Geometry check sheet. Reference: the model listing, model coordinates, mm. Face numbers are marked on the shaded views. A direction names the side the tool comes from. Give positions to 0.01 mm unless a question says otherwise; leave off trailing zeros. Loops run counter-clockwise (first coordinate to the right, second up) from the corner with the lowest first, then second, coordinate; pieces in that order, holes last. Notation, with made-up numbers: (-11, 85.25) -> (-7, 85.25) arc R34 cw to (-7, 120.25) -> close; hole circle Ø3 at (23, 60.25). An arc over 180 degrees is marked (long way). One line per question, with ' | ' between items.
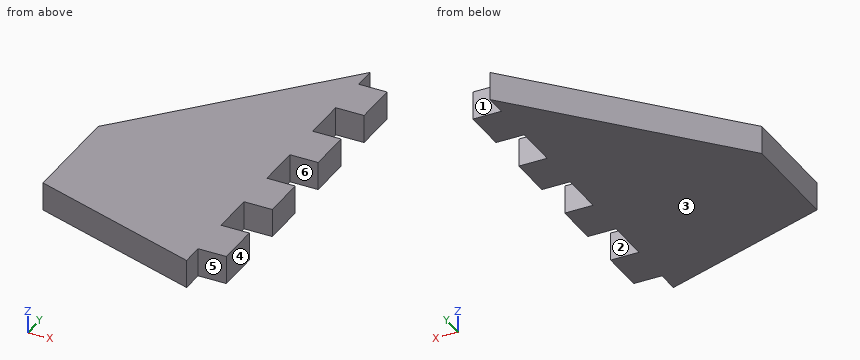
from build123d import *

# Parameters (mm, degrees)
ESTRUSIONE_ESTRUSIONE1_DEPTH = 4
SCHIZZO2_W                   = 4
SCHIZZO2_H                   = 6.25
ESTRUSIONE_ESTRUSIONE2_DEPTH = 4
RIPETIZIONE_A_L1_COUNT       = 4
RIPETIZIONE_A_L1_PITCH       = 12.5


with BuildPart() as part:
    # Schizzo1 → Estrusione-Estrusione1 (new body)
    with BuildSketch(Plane.XY):
        Polygon((-24.4, 23), (-24.4, 8), (0, 0), (0, 50), align=None)
    extrude(amount=ESTRUSIONE_ESTRUSIONE1_DEPTH)

    # Schizzo2 → Estrusione-Estrusione2 (add)
    with BuildSketch(Plane.XY.offset(4)):
        with Locations((2, 43.75)):
            Rectangle(SCHIZZO2_W, SCHIZZO2_H)
    estrusione_estrusione2 = extrude(amount=-ESTRUSIONE_ESTRUSIONE2_DEPTH)

    # Ripetizione a L1: Estrusione-Estrusione2 ×4
    with Locations(*[(0, -i * RIPETIZIONE_A_L1_PITCH, 0) for i in range(1, RIPETIZIONE_A_L1_COUNT)]):
        add(estrusione_estrusione2)


solid = part.part
Item 1: Set-up check for the marked faces 1, 2 and 3: record each of +Z, -Z, +X, -X, +Y, -Y from which the full face is reachable in a straight line by a thin tool's end or side.
Result:
face 1: +Z, -Z, +X, +Y | face 2: +Z, -Z, +X | face 3: -Z, +X, -X, +Y, -Y
Item 2: Depth check by flat-ended pin: pin 1 Ø2 at (y, z) = (37, 0.5) entering from +X; pin 2 Ø2 at (x, z) = (3, 1) entering from -Y (3 decimals); pin 3 Ø1.2 at (x, z) = (2.5, 1) entering from +Y (3 decimals). Enter the tip coordinate at first touch or a pass-through.
Result:
pin 1: x = 0 | pin 2: y = 3.125 | pin 3: y = 46.875
Item 3: Scan lines: probe 1 along Y at (x, z) = (2.25, 0.2) (3 decimals); probe 2 along Y at (x, z) = (-10.75, 3); probe 3 along Y at (x, z) = (-1.25, 1.55). Record each from-to range of solid material in increasing order.
Result:
probe 1: 3.125 to 9.375, 15.625 to 21.875, 28.125 to 34.375, 40.625 to 46.875 | probe 2: 3.52 to 38.1 | probe 3: 0.41 to 48.62
Item 4: Sectioned sample at A-A (z = 0.7). Record the cut outline in (x, y) (3 decimals).
Result:
outline: (-24.4, 8) -> (0, 0) -> (0, 3.125) -> (4, 3.125) -> (4, 9.375) -> (0, 9.375) -> (0, 15.625) -> (4, 15.625) -> (4, 21.875) -> (0, 21.875) -> (0, 28.125) -> (4, 28.125) -> (4, 34.375) -> (0, 34.375) -> (0, 40.625) -> (4, 40.625) -> (4, 46.875) -> (0, 46.875) -> (0, 50) -> (-24.4, 23) -> close
Item 5: Sectioned sample at B-B (y = 11.5). Record the cut outline in (x, z).
Result:
outline: (-24.4, 0) -> (0, 0) -> (0, 4) -> (-24.4, 4) -> close
Item 6: Sectioned sample at C-C (x = -20.75). Record the cut outline in (y, z), plus the area to 3 significant figures.
Result:
outline: (6.8, 0) -> (27.04, 0) -> (27.04, 4) -> (6.8, 4) -> close | area: 80.9 mm2
Item 7: Release check for a two-part mould opening along Y. For the marked faces 4, 5 and 6 record: pulls with the +Y half, pulls with the -Y half, needs draft (parallel to the pull), parting line crosses it, or undercut.
Result:
face 4: needs draft | face 5: pulls with the -Y half | face 6: undercut
